Autodesk Inventor part; units mm, degrees
ref_plane "YZ Plane" through (0, 0, 0) normal (1, 0, 0) x (0, 1, 0)
ref_plane "XZ Plane" through (0, 0, 0) normal (0, 1, 0) x (-1, 0, 0)
ref_plane "XY Plane" through (0, 0, 0) normal (0, 0, 1) x (1, 0, 0)
sketch "Sketch1" plane through (0, 0, 0) normal (0, 0, 1) x (1, 0, 0)
  line L0 (18.5, -19.5) -> (-18.5, -19.5)
  line L1 (-18.5, -19.5) -> (-18.5, 19.5)
  line L2 (-18.5, 19.5) -> (18.5, 19.5)
  line L3 (18.5, 19.5) -> (18.5, -19.5)
  line L4 (18.5, -19.5) -> (-18.5, 19.5) construction
  line L5 (-18.5, -19.5) -> (18.5, 19.5) construction
  circle A0 centre (-2.5, -8.5) radius 9 construction
  circle A1 centre (-8.764, 9.5) radius 9 construction
  circle A2 centre (-15, -9.5) radius 2.5 construction
  circle A3 centre (15, 16) radius 2.5 construction
  circle A4 centre (15, -9.5) radius 2.5 construction
  line L6 (-15, -9.5) -> (15, -9.5) construction
  point P0 (0, 0)
  point P1 (0, -9.5)
  dimension "d0" = 37
  dimension "d1" = 39
  dimension "d2" = 11
  dimension "d3" = 2.5
  dimension "d4" = 18
  dimension "d5" = 18
  dimension "d6" = 18
  dimension "d7" = 6.264
  dimension "d8" = 5
  dimension "d10" = 30
  dimension "d11" = 10
  dimension "d12" = 3.5
  dimension "d13" = 3.5
extrude "Plate1" add sketch "Sketch1" along normal blind 3.048
sketch "Sketch2" plane through (-18.5, -16.452, 3.048) normal (0, -1, 0) x (1, 0, 0)
  line L0 (37, 0) -> (0, 0)
  line L1 (0, 0) -> (0, -20.048)
  line L2 (0, -20.048) -> (37, -20.048)
  line L3 (37, -20.048) -> (37, 0)
edge flange "Flange1" height 17 angle 90 thickness 3.048 bend radius 3.048 thickness toward (0, -1, 0) relief tear relief width 3.048 relief depth 1.524 edges at (0, -19.5, 0) wall of the first edge with corners at (18.5, -16.452, 3.048) (-18.5, -16.452, 3.048) (-18.5, -16.452, -17) (18.5, -16.452, -17)
bend "Bend1"
corner "Corner1"
hole "Hole1" at (-2.5, -8.5, 0) at (-8.764, 9.5, 0) direction (0, 0, 1) diameter 3.3 end through all
hole "Hole2" at (15, 16, 0) at (15, -9.5, 0) at (-15, -9.5, 0) direction (0, 0, 1) diameter 3.3 end through all
sketch "Sketch3" plane through (-18.5, -16.452, -17) normal (0, 1, 0) x (1, 0, 0)
  line L0 (0, -13.952) -> (37, -13.952) construction
  line L1 (37, -13.952) -> (37, 0) construction
  line L2 (37, 0) -> (0, 0) construction
  line L3 (0, -13.952) -> (0, 0) construction
  line L4 (8.5, -8.5) -> (28.5, -8.5) construction
  line L5 (8.5, -8.5) -> (0, -8.5) construction
  line L6 (0, -8.5) -> (0, 0) construction
  line L7 (0, 0) -> (8.5, 0) construction
  line L8 (8.5, 0) -> (8.5, -8.5) construction
  point P0 (18.5, -17)
  point P1 (18.5, 0)
  point P2 (18.5, -8.5)
  dimension "d39" = 20
hole "Hole3" at (-10, -16.452, -8.5) at (10, -16.452, -8.5) direction (0, -1, 0) diameter 5.3 end through all
fillet "Fillet1" radius 2 4 edges at (18.5, -17.976, -17) (-18.5, 19.5, 1.524) (18.5, 19.5, 1.524) (-18.5, -17.976, -17)
ref_plane "Work Plane1" through (0, -16.452, -17) normal (-1, 0, 0) x (0, -1, 0)
equation "\"d13\" = d12"
equation "\"d30\" = Thickness"
equation "\"d14\" = Thickness"
equation "\"d15\" = BendReliefWidth"
equation "\"d16\" = BendReliefDepth"
equation "\"d17\" = MinimumRemnant"
equation "\"d18\" = TransitionRadius"
equation "\"d21\" = BendRadius"
equation "\"d22\" = CornerReliefSize"
equation "\"d23\" = GapSize"
equation "\"d24\" = JacobiRadiusSize"
equation "\"BendRadius\" = Thickness"
equation "\"BendReliefWidth\" = Thickness"
equation "\"BendReliefDepth\" = 0.5 * Thickness"
equation "\"CornerReliefSize\" = 4 * Thickness"
equation "\"MinimumRemnant\" = 2 * Thickness"
equation "\"TransitionRadius\" = BendRadius"
equation "\"JacobiRadiusSize\" = BendRadius"
equation "\"GapSize\" = Thickness"
properties part number "XY Idler Mount"
Source: CAD feature listing. Evaluate the final solid. Frame: model axes, mm. Round coordinates to 2 decimals unless told otherwise and drop trailing zeros. Write each loop counter-clockwise with the first axis right and the second up, starting at its lowest first coordinate (ties: lowest second). Pieces come first, ordered by that corner, then holes. Notation, with made-up numbers: M -11,-7.5 L 12,-7.5 A28 cw 12,11.5 Z; hole C 57,-5.75 d7. An arc over 180 degrees is marked long. One line per item, written item: value. Start each with the question number.
Item 1: Section query B-B (y = 16). Return the cut outline in (x, z).
Item 2: Section query D-D (x = 3). Return the cut outline in (y, z), plus the area to 3 significant figures.
Item 3: Ray query, L1, parallel to X at y = -18.5, z = -8.5; L2, parallel to X at y = 9.5, z = 0.75; L3, parallel to X at y = 16, z = 1.7. Return the intervals inside material, ascending. Write a range as from..to.
Item 4: Section query A-A (z = -8.5). Return the cut outline in (x, y), plus the area to 3 significant figures.
Item 5: Pin query (flat end, axial travel): pin 1 (5.5 mm diameter, centred on x = -8.764, y = 9.5, fed in from +Z); pin 2 (8 mm diameter, centred on x = 8.5, y = 0.5, fed in from -Z); pin 3 (7 mm diameter, centred on x = -4, z = -11.5, fed in from +Y). Return the tip coordinate at first contact, or that it passes through.
Item 6: Mould query, pull axis Y, two halves, no side actions, for faces 1 (the flat face through (0, -16.452, -10)), 2 (the flat face through (0, 3, 0)), 3 (the cylindrical face through (14.504, 17.574, 1.545)), 4 (the cylindrical face through (-0.259, -17.762, 1.215)). Classes: pulls with the +Y half, pulls with the -Y half, needs draft (parallel to the pull), parting line crosses it, or undercut.
Item 7: Section query C-C (x = 15). Return the cut outline in (y, z).
Result set:
1. outline: M -18.5,0 L 13.35,0 L 13.35,3.05 L -18.5,3.05 Z; M 16.65,0 L 18.5,0 L 18.5,3.05 L 16.65,3.05 Z
2. outline: M -19.5,-17 L -16.45,-17 L -16.45,-3.05 A3.05 cw -13.4,0 L 19.5,0 L 19.5,3.05 L -13.4,3.05 A6.1 ccw -19.5,-3.05 Z
2. area: 165 mm²
3. L1: x = -18.5..-12.65, -7.35..7.35, 12.65..18.5
3. L2: x = -18.5..-10.41, -7.11..18.5
3. L3: x = -18.5..13.35, 16.65..18.5
4. outline: M -18.5,-19.5 L -12.65,-19.5 L -12.65,-16.45 L -18.5,-16.45 Z; M -7.35,-19.5 L 7.35,-19.5 L 7.35,-16.45 L -7.35,-16.45 Z; M 12.65,-19.5 L 18.5,-19.5 L 18.5,-16.45 L 12.65,-16.45 Z
4. area: 80.5 mm²
5. pin 1: stops at z = 3.05
5. pin 2: stops at z = 0
5. pin 3: stops at y = -16.45
6. face 1: pulls with the +Y half
6. face 2: needs draft
6. face 3: undercut
6. face 4: pulls with the -Y half
7. outline: M -19.5,-17 L -16.45,-17 L -16.45,-3.05 A3.05 cw -13.4,0 L -11.15,0 L -11.15,3.05 L -13.4,3.05 A6.1 ccw -19.5,-3.05 Z; M -7.85,0 L 14.35,0 L 14.35,3.05 L -7.85,3.05 Z; M 17.65,0 L 19.5,0 L 19.5,3.05 L 17.65,3.05 Z
